```python
from build123d import *

# Parameters (mm, degrees)
CROQUIS1_R              = 135
SALIENTE_EXTRUIR1_DEPTH = 43
REDONDEO5_R             = 20
CROQUIS2_R              = 133
CORTAR_EXTRUIR6_DEPTH   = 25
REDONDEO6_R             = 25
CROQUIS4_R              = 80
CORTAR_EXTRUIR7_DEPTH   = 1
CORTAR_EXTRUIR8_DEPTH   = 67
CROQUIS6_R              = 10
CORTAR_EXTRUIR9_DEPTH   = 1
CORTAR_EXTRUIR10_DEPTH  = 0.5
SALIENTE_EXTRUIR3_DEPTH = 40
SALIENTE_EXTRUIR4_DEPTH = 5
CORTAR_EXTRUIR11_DEPTH  = 5


with BuildPart() as part:
    # Croquis1 → Saliente-Extruir1 (new body)
    with BuildSketch(Plane(origin=(0, 0, 0), x_dir=(1, 0, 0), z_dir=(0, 1, 0))):
        with Locations(Location((0, 0, 0), (0, 0, 270))):
            Circle(CROQUIS1_R)
    extrude(amount=SALIENTE_EXTRUIR1_DEPTH)

    # Redondeo5
    redondeo5_edges = [part.edges().sort_by_distance(p)[0] for p in [
        (0, 43, -135),
    ]]
    fillet(redondeo5_edges, radius=REDONDEO5_R)

    # Croquis2 → Cortar-Extruir6 (cut)
    with BuildSketch(Plane(origin=(0, 0, 0), x_dir=(-1, 0, 0), z_dir=(0, -1, 0))):
        with Locations(Location((0, 0, 0), (0, 0, 90))):
            Circle(CROQUIS2_R)
    extrude(amount=-CORTAR_EXTRUIR6_DEPTH, mode=Mode.SUBTRACT)

    # Redondeo6
    redondeo6_edges = [part.edges().sort_by_distance(p)[0] for p in [
        (0, 25, 133),
    ]]
    fillet(redondeo6_edges, radius=REDONDEO6_R - 0.0001)  # a hair under: the kernel refuses the full size

    # Croquis4 → Cortar-Extruir7 (cut)
    with BuildSketch(Plane(origin=(0, 43, 0), x_dir=(1, 0, 0), z_dir=(0, 1, 0))):
        with Locations(Location((0, 0, 0), (0, 0, 270))):
            Circle(CROQUIS4_R)
    extrude(amount=-CORTAR_EXTRUIR7_DEPTH, mode=Mode.SUBTRACT)

    # Croquis5 → Cortar-Extruir8 (cut)
    with BuildSketch(Plane(origin=(0, 42, 0), x_dir=(1, 0, 0), z_dir=(0, 1, 0))):
        with BuildLine():
            Line((-45, 0), (-45, 40))
            Line((-45, 40), (45, 40))
            Line((45, 40), (45, 0))
            ThreePointArc((45, 0), (0, -20.207972894), (-45, 0))
        make_face()
    extrude(amount=-CORTAR_EXTRUIR8_DEPTH, mode=Mode.SUBTRACT)

    # Croquis6 → Cortar-Extruir9 (cut)
    with BuildSketch(Plane(origin=(0, 43, 0), x_dir=(1, 0, 0), z_dir=(0, 1, 0))):
        with Locations(Location((0, 97.5, 0), (0, 0, 270))):
            Circle(CROQUIS6_R)
    extrude(amount=-CORTAR_EXTRUIR9_DEPTH, mode=Mode.SUBTRACT)

    # Croquis7 → Cortar-Extruir10 (cut)
    with BuildSketch(Plane(origin=(0, 42, 0), x_dir=(1, 0, 0), z_dir=(0, 1, 0))):
        with BuildLine():
            Line((-1, 97.5), (-1, 104.846686009))
            ThreePointArc((-1, 104.846686009), (0, 105.846686009), (1, 104.846686009))
            Line((1, 104.846686009), (1, 97.5))
            ThreePointArc((1, 97.5), (0, 96.5), (-1, 97.5))
        make_face()
        with BuildLine():
            ThreePointArc((-3.025522609, 103.54170716), (0.056423139, 90.743312284), (2.924202621, 103.591391589))
            ThreePointArc((2.924202621, 103.591391589), (2.037712876, 103.279966687), (2.349137778, 102.393476942))
            ThreePointArc((2.349137778, 102.393476942), (0.045327135, 92.072062056), (-2.430532483, 102.353563302))
            ThreePointArc((-2.430532483, 102.353563302), (-2.133955617, 103.245130294), (-3.025522609, 103.54170716))
        make_face()
    extrude(amount=-CORTAR_EXTRUIR10_DEPTH, mode=Mode.SUBTRACT)



with BuildPart() as body_2:
    # Croquis9 → Saliente-Extruir3 (new body)
    with BuildSketch(Plane.XZ.offset(-25)):
        with BuildLine():
            Line((45, -40), (-45, -40))
            Line((-45, -40), (-45, 0))
            ThreePointArc((-45, 0), (0, 20.207972894), (45, 0))
            Line((45, 0), (45, -40))
        make_face()
        with BuildLine():
            Line((44, -39), (-44, -39))
            Line((-44, -39), (-44, -0.382023598))
            ThreePointArc((-44, -0.382023598), (0, 19.207972894), (44, -0.382023598))
            Line((44, -0.382023598), (44, -39))
        make_face(mode=Mode.SUBTRACT)
    extrude(amount=SALIENTE_EXTRUIR3_DEPTH)


with BuildPart() as part_1:
    add(part.part)

    add(body_2.part)  # Saliente-Extruir4 merges body 2
    # Croquis11 → Saliente-Extruir4 (add)
    with BuildSketch(Plane.XZ.offset(-25)):
        with BuildLine():
            Line((47, -42), (47, 0.753305284))
            ThreePointArc((47, 0.753305284), (0, 22.207972894), (-47, 0.753305284))
            Line((-47, 0.753305284), (-47, -42))
            Line((-47, -42), (47, -42))
        make_face()
        with BuildLine():
            Line((45, 0), (45, -40))
            Line((45, -40), (-45, -40))
            Line((-45, -40), (-45, 0))
            ThreePointArc((-45, 0), (0, 20.207972894), (45, 0))
        make_face(mode=Mode.SUBTRACT)
    extrude(amount=SALIENTE_EXTRUIR4_DEPTH)

    # Croquis12 → Cortar-Extruir11 (cut)
    with BuildSketch(Plane(origin=(0, 42, 0), x_dir=(1, 0, 0), z_dir=(0, 1, 0))):
        with BuildLine():
            Line((47, -0.753305284), (47, 42))
            Line((47, 42), (-47, 42))
            Line((-47, 42), (-47, -0.753305284))
            ThreePointArc((-47, -0.753305284), (0, -22.207972894), (47, -0.753305284))
        make_face()
        with BuildLine():
            Line((45, 40), (-45, 40))
            Line((-45, 40), (-45, 0))
            ThreePointArc((-45, 0), (0, -20.207972894), (45, 0))
            Line((45, 0), (45, 40))
        make_face(mode=Mode.SUBTRACT)
    extrude(amount=-CORTAR_EXTRUIR11_DEPTH, mode=Mode.SUBTRACT)


solid = part_1.part
```
Source: CAD feature listing. Evaluate the final solid. Frame: model axes, mm. A direction names the side the tool comes from. Give positions to 0.01 mm unless a question says otherwise; leave off trailing zeros. Write each loop counter-clockwise with the first axis right and the second up, starting at its lowest first coordinate (ties: lowest second). Pieces come first, ordered by that corner, then holes.
1. Material intervals for line 1 along X through (y, z) = (-2.5, -11); line 2 along Y through (x, z) = (-33.5, 97.5); line 3 along Z through (x, y) = (35.5, 10), sorted ascending.
2. Section query A-A (y = 9). Return the cut outline in (x, z).
3. First-contact query: pin 1 (1 mm diameter, centred on x = -34.5, y = -6, fed in from -Z); pin 2 (4 mm diameter, centred on x = 65, z = -65.5, fed in from -Y); pin 3 (5 mm diameter, centred on y = 21.5, z = -81.5, fed in from -X). Flat tips, straight axial feed; report the tip coordinate or a pass-through.
4. Pull-direction query (Z, two-part tool) for faces 1 (the face through (-0.746, 39.535, 22.204)), 2 (the face through (7, -15, 19)); classes: +Z half, -Z half, draft (parallel to the pull), parting line (faces both ways), or undercut.
5. Access query for faces 3 (the face through (-44, 5, -20)), 4 (the face through (-78.1, 42.51, -17.34)), 5 (the face through (-0.712, 2.745, 20.204)), 6 (the face through (78, 43, 24)). Directions: +Z, -Z, +X, -X, +Y, -Y. A direction counts if a zero-diameter tool reaches every point of the face in a straight line with its end or side. Return the directions, or none.
Output values:
1. line 1: x = -45 to -44, 44 to 45
1. line 2: y = 25 to 43
1. line 3: z = -130.25 to -126.01, -40 to -39, 7.38 to 8.63, 126.01 to 130.25
2. outline: circle Ø270 at (0, 0); (-45, -40) - (45, -40) - (45, 0) arc R60.21 ccw to (-45, 0) - close; hole circle Ø262.65 at (0, 0); hole (-44, -39) - (44, -39) - (44, -0.38) arc R59.21 ccw to (-44, -0.38) - close
3. pin 1: stops at z = -40
3. pin 2: stops at y = 25
3. pin 3: stops at x = -109.47
4. face 1: undercut
4. face 2: draft
5. face 3: +Y, -Y
5. face 4: +Y
5. face 5: -Y
5. face 6: +Z, -Z, +X, -X, +Y
